Check sheet for the modelled part. Datum: model origin and axes. Units: mm. A direction names the side the tool comes from. Round coordinates to 2 decimals unless told otherwise and drop trailing zeros. Write each loop counter-clockwise with the first axis right and the second up, starting at its lowest first coordinate (ties: lowest second). Pieces come first, ordered by that corner, then holes.
from build123d import *

# Parameters (mm, degrees)
SKETCH1_W           = 326.39
SKETCH1_H           = 60.799999812
BOSS_EXTRUDE1_DEPTH = 5
SKETCH9_W           = 16.959219297
SKETCH9_H           = 5.08
CUT_EXTRUDE2_DEPTH  = 5.08
CUT_EXTRUDE3_REACH  = 333.163
SKETCH11_W          = 5
SKETCH11_H          = 10.254787301


with BuildPart() as part:
    # Sketch1 → Boss-Extrude1 (new body)
    with BuildSketch(Plane.XY):
        with Locations((-163.195, 25.4)):
            Rectangle(SKETCH1_W, SKETCH1_H)
    extrude(amount=BOSS_EXTRUDE1_DEPTH)

    # Sketch9 → Cut-Extrude2 (cut)
    with BuildSketch(Plane.XY.offset(4.999999906)):
        with Locations((-46.614250443, -2.459999906)):
            Rectangle(SKETCH9_W, SKETCH9_H)
        with Locations((-8.479609649, -2.459999906)):
            Rectangle(SKETCH9_W, SKETCH9_H)
        with Locations((-8.479609649, 53.259999906)):
            Rectangle(SKETCH9_W, SKETCH9_H)
        with Locations((-46.614250443, 53.259999906)):
            Rectangle(SKETCH9_W, SKETCH9_H)
        with Locations((-279.775749558, 53.259999906)):
            Rectangle(SKETCH9_W, SKETCH9_H)
        with Locations((-317.910390352, 53.259999906)):
            Rectangle(SKETCH9_W, SKETCH9_H)
        with Locations((-317.910390352, -2.459999906)):
            Rectangle(SKETCH9_W, SKETCH9_H)
        with Locations((-279.775749558, -2.459999906)):
            Rectangle(SKETCH9_W, SKETCH9_H)
    extrude(amount=-CUT_EXTRUDE2_DEPTH, mode=Mode.SUBTRACT)

    # Sketch11 → Cut-Extrude3 (cut, up to next)
    with BuildSketch(Plane(origin=(0, 0, 0), x_dir=(-1, 0, 0), z_dir=(0, 0, -1)), mode=Mode.PRIVATE) as cut_extrude3_sk1:
        with Locations((8.85, 37.976893645)):
            Rectangle(SKETCH11_W, SKETCH11_H)
    cut_extrude3_tool1 = extrude(cut_extrude3_sk1.sketch, amount=-CUT_EXTRUDE3_REACH, mode=Mode.PRIVATE) & part.part
    # Sketch11 → Cut-Extrude3 (cut, up to next)
    with BuildSketch(Plane(origin=(0, 0, 0), x_dir=(-1, 0, 0), z_dir=(0, 0, -1)), mode=Mode.PRIVATE) as cut_extrude3_sk2:
        with Locations((8.85, 12.743106261)):
            Rectangle(SKETCH11_W, SKETCH11_H)
    cut_extrude3_tool2 = extrude(cut_extrude3_sk2.sketch, amount=-CUT_EXTRUDE3_REACH, mode=Mode.PRIVATE) & part.part
    # Sketch11 → Cut-Extrude3 (cut, up to next)
    with BuildSketch(Plane(origin=(0, 0, 0), x_dir=(-1, 0, 0), z_dir=(0, 0, -1)), mode=Mode.PRIVATE) as cut_extrude3_sk3:
        with Locations((317.54, 12.743106261)):
            Rectangle(SKETCH11_W, SKETCH11_H)
    cut_extrude3_tool3 = extrude(cut_extrude3_sk3.sketch, amount=-CUT_EXTRUDE3_REACH, mode=Mode.PRIVATE) & part.part
    # Sketch11 → Cut-Extrude3 (cut, up to next)
    with BuildSketch(Plane(origin=(0, 0, 0), x_dir=(-1, 0, 0), z_dir=(0, 0, -1)), mode=Mode.PRIVATE) as cut_extrude3_sk4:
        with Locations((317.54, 37.976893645)):
            Rectangle(SKETCH11_W, SKETCH11_H)
    cut_extrude3_tool4 = extrude(cut_extrude3_sk4.sketch, amount=-CUT_EXTRUDE3_REACH, mode=Mode.PRIVATE) & part.part
    add(cut_extrude3_tool1.solids().sort_by_distance((-8.85, 37.976894, 0))[0], mode=Mode.SUBTRACT)
    add(cut_extrude3_tool2.solids().sort_by_distance((-8.85, 12.743106, 0))[0], mode=Mode.SUBTRACT)
    add(cut_extrude3_tool3.solids().sort_by_distance((-317.54, 12.743106, 0))[0], mode=Mode.SUBTRACT)
    add(cut_extrude3_tool4.solids().sort_by_distance((-317.54, 37.976894, 0))[0], mode=Mode.SUBTRACT)


solid = part.part
1. Sectioned sample at B-B, the plane z = 4.1. Give the number of separate pieces and of enclosed holes in the cut face, plus the area to 3 significant figures.
2. Set-up check for faces 4 (the flat face through (-6.35, 38, 2)), 5 (the flat face through (-16.959, 53, 3)), 6 (the flat face through (-271.296, 53, 3)): record each of +Z, -Z, +X, -X, +Y, -Y from which the full face is reachable in a straight line by a thin tool's end or side.
3. Go/stop test with flat-tipped pins: pin 1 (2.5 mm diameter, centred on x = -316.5, z = 2, fed in from +Y); pin 2 (2.5 mm diameter, centred on x = -9.5, z = 1.5, fed in from -Y). Record where each tip stops, or that it passes through.
4. Release check for a two-part mould opening along X. For faces 1 (the flat face through (0, 25, 2)), 2 (the flat face through (-28, -5, 2)), 3 (the flat face through (-47, 50.72, 3)) record: released by +X, released by -X, zero draft, split by the parting line, or undercut.
5. Scan lines: line 1 along X through (y, z) = (37, 3.5); line 2 along Y through (x, z) = (-38.5, 3.2). Record each from-to range of solid material in increasing order.
6. Sectioned sample at A-A, the plane y = 36.5. Enter the section's corners in (x, z).
Computed values:
1. separate pieces: 1
1. enclosed holes: 4
1. area: 19,000 mm2
2. face 4: +Z, -Z
2. face 5: +Z, -Z, +X, +Y
2. face 6: +Z, -Z, +Y
3. pin 1: stops at y = 50.72
3. pin 2: stops at y = 0.08
4. face 1: released by +X
4. face 2: zero draft
4. face 3: undercut
5. line 1: x = -326.39 to -320.04, -315.04 to -11.35, -6.35 to 0
5. line 2: y = 0.08 to 50.72
6. outline: (-326.39, 0) - (-320.04, 0) - (-320.04, 5) - (-326.39, 5) - close; (-315.04, 0) - (-11.35, 0) - (-11.35, 5) - (-315.04, 5) - close; (-6.35, 0) - (0, 0) - (0, 5) - (-6.35, 5) - close
